Input: dimensioned drawing with shaded views. Units: mm. Origin: part minimum x, y, z. A direction names the side the tool comes from. Coordinates: 2 decimals unless noted, no trailing zeros. Loops run counter-clockwise (first coordinate to the right, second up) from the corner with the lowest first, then second, coordinate; pieces in that order, holes last.
(1) Section B-B, the plane z = 87. Return loops of the section in (x, y), then the cut area to 3 significant figures.
(2) Section D-D, the plane x = 107. Return loops of the section in (y, z), then the cut area to 3 significant figures.
(3) Section C-C, the plane y = 48. Return loops of the section in (x, z).
(4) Set-up query: the marked faces 3, 4, 5, 6 and 7. Return all of +Z, -Z, +X, -X, +Y, -Y with unobstructed straight access to the full face (end or side cutting, diameter ignored); none if empty.
(5) Line query: L1, parallel to Z at x = 86, y = 18.5; L2, parallel to Y at x = 80, z = 158.45 (1 decimal); L3, parallel to Y at x = 80, z = 3.55. Output: solid intervals per line, ascending.
(6) Section A-A, the plane y = 31. Return loops of the section in (x, z).
(7) Mould query, pull axis X, two halves, no side actions, for the marked faces 1 and 2. Classes: released by +X, released by -X, zero draft, split by the parting line, or undercut.
(8) Contact query for flat-ended pins moving along their axis: P1, Ø20, axis at x = 119, y = 54, coming from the +Z side; P2, Ø10, axis at y = 50.5, z = 37.5, coming from the -X side; P3, Ø18, axis at y = 27.5, z = 141.5, coming from the -X side; P4, Ø20, axis at x = 15, y = 56, coming from the -Z side. Output: stop coordinate, or through.
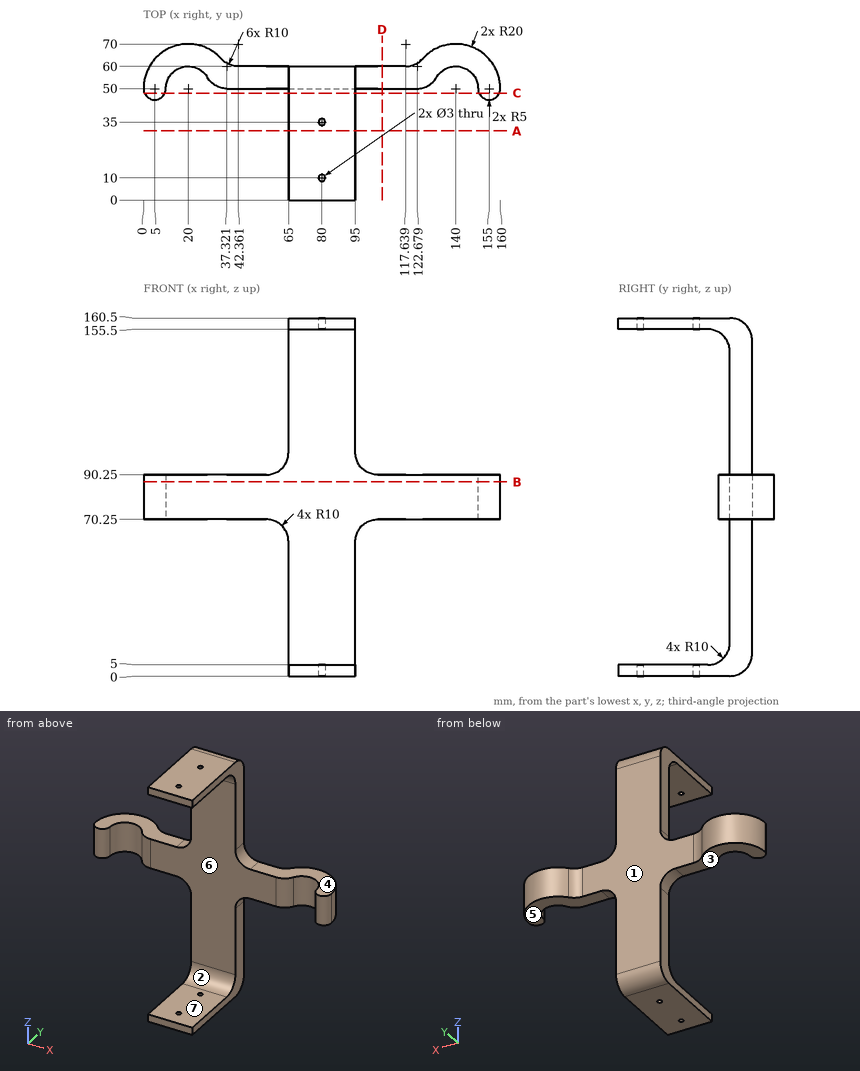
Report:
1. outline: (0, 50) arc R5 ccw to (10, 50) arc R10 cw to (28.66, 55) arc R10 ccw to (37.32, 50) - (122.68, 50) arc R10 ccw to (131.34, 55) arc R10 cw to (150, 50) arc R5 ccw to (160, 50) arc R20 ccw to (125.09, 63.33) arc R10 cw to (117.64, 60) - (42.36, 60) arc R10 cw to (34.91, 63.33) arc R20 ccw to start
1. area: 1,830 mm2
2. outline: (50, 70.25) - (60, 70.25) - (60, 90.25) - (50, 90.25) - close
2. area: 200 mm2
3. outline: (0.42, 70.25) - (9.58, 70.25) - (9.58, 90.25) - (0.42, 90.25) - close; (65, 0) - (95, 0) - (95, 9) - (65, 9) - close; (65, 151.5) - (95, 151.5) - (95, 160.5) - (65, 160.5) - close; (150.42, 70.25) - (159.58, 70.25) - (159.58, 90.25) - (150.42, 90.25) - close
4. face 3: -Z, -X, +Y, -Y
4. face 4: +Z, +X, +Y, -Y
4. face 5: -Z, +X, +Y, -Y
4. face 6: -Y
4. face 7: +X, -X, -Y
5. L1: z = 0 to 5, 155.5 to 160.5
5. L2: y = 0 to 8.5, 11.5 to 33.5, 36.5 to 56.1
5. L3: y = 0 to 8.5, 11.5 to 33.5, 36.5 to 57.64
6. outline: (65, 0) - (95, 0) - (95, 5) - (65, 5) - close; (65, 155.5) - (95, 155.5) - (95, 160.5) - (65, 160.5) - close
7. face 1: undercut
7. face 2: zero draft
8. P1: stops at z = 90.25
8. P2: stops at x = 65
8. P3: passes through
8. P4: stops at z = 70.25
